from build123d import *

# Parameters (mm, degrees)
ESQUISSE2_R      = 2
EXTRUSION1_DEPTH = 32


with BuildPart() as part:
    # Esquisse1 → Révolution1 (revolve)
    with BuildSketch(Plane.XY):
        Polygon((0, 10), (0, 17.5), (5, 17.5), (5, 11), (31, 11), (31, 6.5), (20, 6.5), (20, 10), align=None)
    revolve(axis=Axis((0, 0, 0), (1, 0, 0)))

    # Esquisse2 → Extrusion1 (cut, through all)
    with BuildSketch(Plane.ZY):
        with Locations((0, 15)):
            Circle(ESQUISSE2_R)
        with Locations((15, 0)):
            Circle(ESQUISSE2_R)
        with Locations((0, -15)):
            Circle(ESQUISSE2_R)
        with Locations((-15, 0)):
            Circle(ESQUISSE2_R)
    extrude(amount=-EXTRUSION1_DEPTH, mode=Mode.SUBTRACT)


solid = part.part
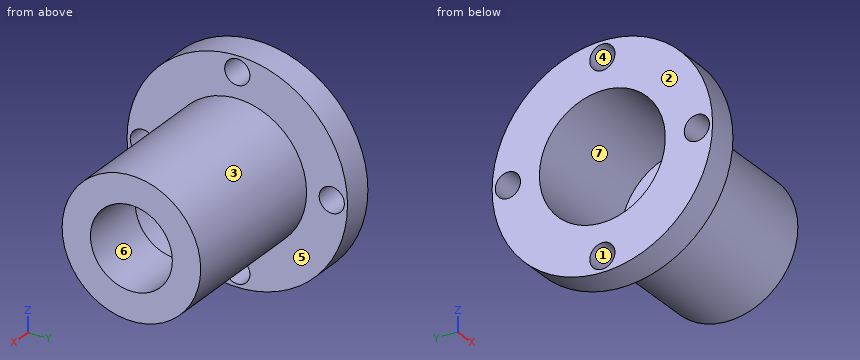
Input: part model. Units: mm. Frame: model coordinates. Face numbers are marked on the shaded views. A direction names the side the tool comes from. Round coordinates to 2 decimals unless told otherwise and drop trailing zeros. Order: outer loops, then holes, each group sorted by start corner. A loop starts at its lowest first (then second) coordinate and runs counter-clockwise, first axis right, second up. Notation, with made-up numbers: (-30.5, 24.5) - (9.5, 24.5) arc R23 cw to (9.5, 36.5) - close; hole circle Ø4 at (-12, 10.5). An arc over 180 degrees is marked (long way). Answer as a JSON object with one key per item and string values. Group by question number.
(1) Cut plane A-A (z = 0). Return loops of the section in (x, y).
(2) Reachability of the marked faces 5, 6 and 7 from +Z, -Z, +X, -X, +Y, -Y: full face, straight path, thin tool, end or side. Return the list, or none.
(3) Cut plane C-C (y = -3.5). Return loops of the section in (x, z), then the cut area to 3 significant figures.
(4) Draft query along Y for the marked faces 1, 2, 3 and 4. Return one class per face: released by +Y, released by -Y, zero draft, split by the parting line, or undercut.
(5) Material intervals for probe 1 along Z at (x, y) = (27.75, 0); probe 2 along X at (y, z) = (12, 10); probe 3 along Y at (x, z) = (16.5, -6.5), sorted ascending. Write a range as from..to.
(6) Pin query (flat end, axial travel): P1, Ø2.5, axis at y = 0, z = -15, coming from the +X side; P2, Ø12, axis at x = 9.5, z = 0, coming from the -Y side; P3, Ø8, axis at x = 15, z = -2, coming from the -Y side; P4, Ø1, axis at y = 10, z = -8, coming from the +X side. Return the tip coordinate at first contact, or that it passes through.
(7) Cut plane D-D (x = 2). Return loops of the section in (y, z), then the cut area to 3 significant figures.
Here are the results:
{
 "1": {"outline": "(0, -17.5) - (5, -17.5) - (5, -17) - (0, -17) - close; (0, -13) - (5, -13) - (5, -11) - (31, -11) - (31, -6.5) - (20, -6.5) - (20, -10) - (0, -10) - close; (0, 10) - (20, 10) - (20, 6.5) - (31, 6.5) - (31, 11) - (5, 11) - (5, 13) - (0, 13) - close; (0, 17) - (5, 17) - (5, 17.5) - (0, 17.5) - close"},
 "2": {"face 5": "+X", "face 6": "+X, -X", "face 7": "-X"},
 "3": {"outline": "(0, -17.15) - (5, -17.15) - (5, -10.43) - (31, -10.43) - (31, -5.48) - (20, -5.48) - (20, -9.37) - (0, -9.37) - close; (0, 9.37) - (20, 9.37) - (20, 5.48) - (31, 5.48) - (31, 10.43) - (5, 10.43) - (5, 17.15) - (0, 17.15) - close", "area": "219 mm^2"},
 "4": {"face 1": "undercut", "face 2": "zero draft", "face 3": "split by the parting line", "face 4": "undercut"},
 "5": {"probe 1": "z = -11..-6.5, 6.5..11", "probe 2": "x = 0..5", "probe 3": "y = -8.87..-7.6, 7.6..8.87"},
 "6": {"P1": "passes through", "P2": "stops at y = -17.5", "P3": "stops at y = -11", "P4": "stops at x = 5"},
 "7": {"outline": "circle Ø35 at (0, 0); hole circle Ø4 at (-15, 0); hole circle Ø20 at (0, 0); hole circle Ø4 at (0, -15); hole circle Ø4 at (0, 15); hole circle Ø4 at (15, 0)", "area": "598 mm^2"}
}
